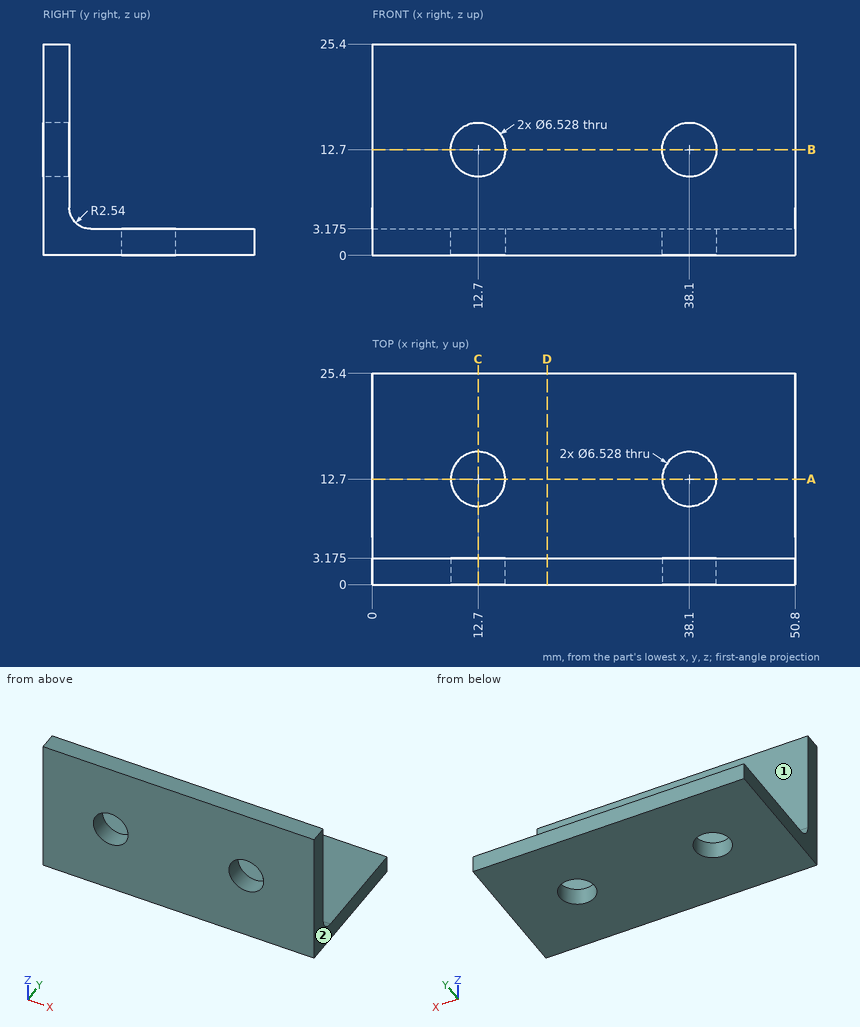
Part print with two shaded views. Sizes in mm from the minimum x, y, z corner. A direction names the side the tool comes from. Coordinates: 2 decimals unless noted, no trailing zeros. Write each loop counter-clockwise with the first axis right and the second up, starting at its lowest first coordinate (ties: lowest second). Pieces come first, ordered by that corner, then holes. Notation, with made-up numbers: (32, 20.5) - (88, 20.5) arc R29 cw to (88, 41.5) - close; hole circle Ø4 at (55.25, -32). An arc over 180 degrees is marked (long way). Use a Markdown table: item, result. Add a question column.
Item 1: Drill centre lines: line 1 along X through (y, z) = (1.3, 12.7); line 2 along Y through (x, z) = (38.1, 1.75). Where is each one in solid material? Low to high.
Item 2: Band-saw the part on D-D, the plane x = 21. Write the cut outline in (y, z) (3 decimals).
Item 3: Band-saw the part on C-C, the plane x = 12.7. Write the cut outline in (y, z) (1 decimal), and give its area (3 significant figures).
Item 4: Band-saw the part on A-A, the plane y = 12.7. Write the cut outline in (x, z) (1 decimal), and give its area (3 significant figures).
Item 5: 3-axis set-ups, long thin cutter, end or side, ignore diameter. For the marked faces 1 and 2: which of +Z, -Z, +X, -X, +Y, -Y reach the whole face in a straight line?
Item 6: Drop flat-ended pins along their axis: pin 1 (10.5 mm diameter, centred on x = 38.1, z = 12.7, fed in from +Y) (3 decimals); pin 2 (6 mm diameter, centred on x = 15.5, y = 19, fed in from +Z) (3 decimals); pin 3 (4 mm diameter, centred on x = 37, y = 5.5, fed in from +Z). Give the stop position or say it passes through.
A:
| question | item | result |
|---|---|---|
| 1 | line 1 | x = 0 to 9.44, 15.96 to 34.84, 41.36 to 50.8 |
| 1 | line 2 | y = 0 to 9.44, 15.96 to 25.4 |
| 2 | outline | (0, 0) - (25.4, 0) - (25.4, 3.175) - (5.715, 3.175) arc R2.54 cw to (3.175, 5.715) - (3.175, 25.4) - (0, 25.4) - close |
| 3 | outline | (0, 0) - (9.4, 0) - (9.4, 3.2) - (5.7, 3.2) arc R2.5 cw to (3.2, 5.7) - (3.2, 9.4) - (0, 9.4) - close; (0, 16) - (3.2, 16) - (3.2, 25.4) - (0, 25.4) - close; (16, 0) - (25.4, 0) - (25.4, 3.2) - (16, 3.2) - close |
| 3 | area | 111 mm² |
| 4 | outline | (0, 0) - (9.4, 0) - (9.4, 3.2) - (0, 3.2) - close; (16, 0) - (34.8, 0) - (34.8, 3.2) - (16, 3.2) - close; (41.4, 0) - (50.8, 0) - (50.8, 3.2) - (41.4, 3.2) - close |
| 4 | area | 120 mm² |
| 5 | face 1 | +Z, +X, -X, +Y |
| 5 | face 2 | +Z, -Z, +X, +Y, -Y |
| 6 | pin 1 | stops at y = 3.175 |
| 6 | pin 2 | stops at z = 3.175 |
| 6 | pin 3 | stops at z = 4.47 |
